Model file for the job. Use its own axes, mm. A direction names the side the tool comes from. Coordinates: 2 decimals unless noted, no trailing zeros. Order: outer loops, then holes, each group sorted by start corner. A loop starts at its lowest first (then second) coordinate and runs counter-clockwise, first axis right, second up. Notation, with made-up numbers: (80, 51) -> (137, 51) arc R19 cw to (137, 72) -> close; hole circle Ø11 at (-15.75, 52). An arc over 180 degrees is marked (long way). Use CSV: the item, a comma, the result in double quotes. Start each with the question number.
(1) Probe L1, parallel to Z at x = 69.5, y = -108; L2, parallel to X at y = -120, z = -112.5; L3, parallel to Z at x = -43.5, y = -189. List the from-to ranges inside material, lowest first.
(2) Tool access for faces 1 (the flat face through (106, -130, -223)), 2 (the flat face through (-1.484, -182.877, -190.464)), 3 (the flat face through (-1.4, -176.89, -192.48)): list every direction of +Z, -Z, +X, -X, +Y, -Y with a clear straight run to the whole face (end or side of a thin tool).
(3) Cut at C-C on y = -116.5. Write the cut outline in (x, z).
(4) Pin check, flat tips, straight feed: pin 1 Ø11 at (x, z) = (5, -382) entering from -Y; pin 2 Ø2.5 at (x, z) = (110, -65.5) entering from -Y; pin 3 Ø6 at (x, z) = (4, -255.5) entering from +Y. Stop position of each tip, or through.
(5) Pull direction Z, two halves, no side cores. Call faces 4 (the flat face through (-106, -130, -223)), 5 (the cylindrical face through (-1.484, -213.599, -230.624)), 6 (the flat face through (-2, -132, -406)): pulls with the +Z half, pulls with the -Z half, needs draft (parallel to the pull), parting line crosses it, or undercut.
(6) Cut at D-D on x = 17. Write the cut outline in (y, z), plus the area to 3 significant figures.
(7) Cut at A-A on y = -186.5. Write the cut outline in (x, z), plus the area to 3 significant figures.
(8) Cut at B-B on z = -380. Write the cut outline in (x, y).
```python
from build123d import *

# Parameters (mm, degrees)
PAN_START            = -106
PAN_BODY_DEPTH       = 212
PAN_START_2          = -406
SKETCH2_W            = 228
SKETCH2_H            = 8
PAN_RAIL_DEPTH       = 478
SUMP_START           = -100
SUMP_DEPTH           = 200
DRAIN_START          = -225
SKETCH4_R            = 11
DRAIN_PLUG_DEPTH     = 11
FILTER_START         = -160
SKETCH5_R            = 42
FILTER_ADAPTER_DEPTH = 11
OIL_START            = -262
SKETCH6_R            = 38
OIL_FILTER_DEPTH     = 102


with BuildPart() as part:
    # Sketch1 → Pan Body (new body)
    with BuildSketch(Plane(origin=(0, 0, 0), x_dir=(0, 0, -1), z_dir=(1, 0, 0)).offset(PAN_START)):
        with BuildLine():
            Line((-72, -70), (406, -70))
            Line((406, -70), (406, -195))
            ThreePointArc((406, -195), (400.142135624, -209.142135624), (386, -215))
            Line((386, -215), (238.876015631, -215))
            ThreePointArc((238.876015631, -215), (230.51154464, -213.559194066), (223.111200004, -209.402850003))
            Line((223.111200004, -209.402850003), (156.888799996, -155.597149997))
            ThreePointArc((156.888799996, -155.597149997), (149.48845536, -151.440805934), (141.123984369, -150))
            Line((141.123984369, -150), (-52, -150))
            ThreePointArc((-52, -150), (-66.142135624, -144.142135624), (-72, -130))
            Line((-72, -130), (-72, -70))
        make_face()
    extrude(amount=PAN_BODY_DEPTH)

    # Sketch2 → Pan Rail (add)
    with BuildSketch(Plane.XY.offset(PAN_START_2)):
        with Locations((0, -74)):
            Rectangle(SKETCH2_W, SKETCH2_H)
    extrude(amount=PAN_RAIL_DEPTH)

    # Sketch3 → Sump (cut)
    with BuildSketch(Plane(origin=(0, 0, 0), x_dir=(0, 0, -1), z_dir=(1, 0, 0)).offset(SUMP_START)):
        with BuildLine():
            Line((-66, -60), (400, -60))
            Line((400, -60), (400, -195))
            ThreePointArc((400, -195), (395.899494937, -204.899494937), (386, -209))
            Line((386, -209), (239.100812505, -209))
            ThreePointArc((239.100812505, -209), (232.409235712, -207.847355253), (226.488960003, -204.522280002))
            Line((226.488960003, -204.522280002), (157.511039997, -148.477719998))
            ThreePointArc((157.511039997, -148.477719998), (151.590764288, -145.152644747), (144.899187495, -144))
            Line((144.899187495, -144), (-52, -144))
            ThreePointArc((-52, -144), (-61.899494937, -139.899494937), (-66, -130))
            Line((-66, -130), (-66, -60))
        make_face()
    extrude(amount=SUMP_DEPTH, mode=Mode.SUBTRACT)

    # Sketch4 → Drain Plug (add)
    with BuildSketch(Plane(origin=(0, 0, 0), x_dir=(1, 0, 0), z_dir=(0, 1, 0)).offset(DRAIN_START)):
        with Locations(Location((0, 380, 0), (0, 0, 146.944268849))):
            Circle(SKETCH4_R)
    extrude(amount=DRAIN_PLUG_DEPTH)

    # Sketch5 → Filter Adapter (add)
    with BuildSketch(Plane(origin=(0, 0, 0), x_dir=(1, 0, 0), z_dir=(0, 1, 0)).offset(FILTER_START)):
        with Locations(Location((-45, 0, 0), (0, 0, 270))):
            Circle(SKETCH5_R)
    extrude(amount=FILTER_ADAPTER_DEPTH)

    # Sketch6 → Oil Filter (add)
    with BuildSketch(Plane(origin=(0, 0, 0), x_dir=(1, 0, 0), z_dir=(0, 1, 0)).offset(OIL_START)):
        with Locations(Location((-45, 0, 0), (0, 0, 270))):
            Circle(SKETCH6_R)
    extrude(amount=OIL_FILTER_DEPTH)


solid = part.part
```
Outcome:
1,L1,"-406 to -400, 66 to 72"
1,L2,"-106 to -100, 100 to 106"
1,L3,"-406 to -400, -207.38 to -198, -37.97 to 37.97"
2,face 1,"+Z, -Z, +X, -Y"
2,face 2,"+X, -X, -Y"
2,face 3,"+Y"
3,outline,"(-106, -406) -> (106, -406) -> (106, 72) -> (-106, 72) -> close; hole (-100, -400) -> (100, -400) -> (100, 66) -> (-100, 66) -> close"
4,pin 1,"y = -225"
4,pin 2,"y = -78"
4,pin 3,"y = -209"
5,face 4,"needs draft"
5,face 5,"undercut"
5,face 6,"pulls with the -Z half"
6,outline,"(-215, -386) arc R20 ccw to (-195, -406) -> (-70, -406) -> (-70, -400) -> (-195, -400) arc R14 cw to (-209, -386) -> (-209, -239.1) arc R20 cw to (-204.52, -226.49) -> (-148.48, -157.51) arc R20 ccw to (-144, -144.9) -> (-144, 52) arc R14 cw to (-130, 66) -> (-70, 66) -> (-70, 72) -> (-130, 72) arc R20 ccw to (-150, 52) -> (-150, -141.12) arc R25 cw to (-155.6, -156.89) -> (-209.4, -223.11) arc R25 ccw to (-215, -238.88) -> close"
6,area,"4,190 mm2"
7,outline,"(-106, -406) -> (106, -406) -> (106, -194.92) -> (-106, -194.92) -> close; circle Ø76 at (-45, 0); hole (-100, -400) -> (100, -400) -> (100, -204.31) -> (-100, -204.31) -> close"
7,area,"10,100 mm2"
8,outline,"(-114, -78) -> (-106, -78) -> (-106, -215) -> (-11, -215) -> (-11, -225) -> (11, -225) -> (11, -215) -> (106, -215) -> (106, -78) -> (114, -78) -> (114, -70) -> (100, -70) -> (100, -209) -> (-100, -209) -> (-100, -70) -> (-114, -70) -> close"
